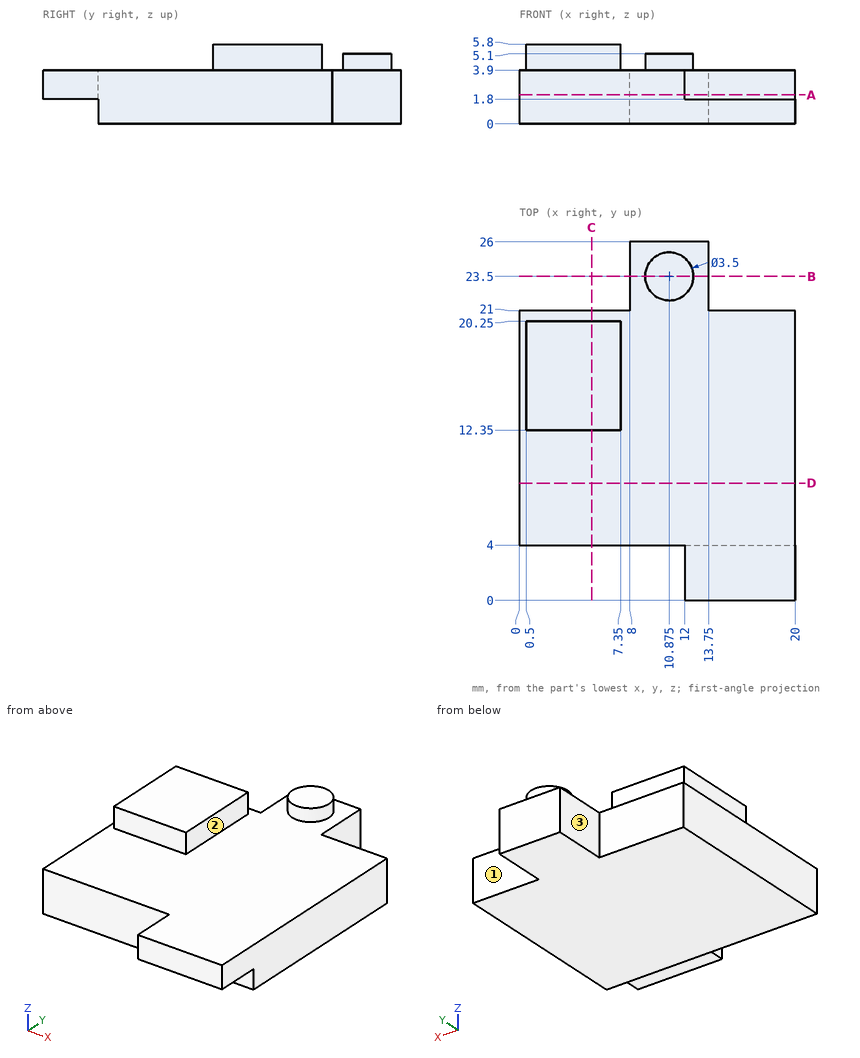
Answer from the drawing. Dimensions are ordinates in mm from the lowest x, y and z of the part. A direction names the side the tool comes from. Give positions to 0.01 mm unless a question says otherwise; leave off trailing zeros. Write each loop counter-clockwise with the first axis right and the second up, starting at its lowest first coordinate (ties: lowest second). Pieces come first, ordered by that corner, then holes. Notation, with made-up numbers: (48, 21.25) - (103, 21.25) arc R18 ccw to (103, 28.25) - close; hole circle Ø10 at (8, 80). An arc over 180 degrees is marked (long way). One line per item, written item: value. Start each with the question number.
1. For the marked faces 1, 2 and 3, determine the directions among +Z, -Z, +X, -X, +Y, -Y from which every point of the face is accessible in a straight line to the end or side of a thin tool.
2. Find section A-A (z = 2.1). Write down the section's boundary in (x, y), then the cut area to 3 significant figures.
3. Find section C-C (x = 5.25). Write down the section's boundary in (y, z), then the cut area to 3 significant figures.
4. Given pin 1 (1.2 mm diameter, centred on x = 3, z = 1.5, fed in from +Y); pin 2 (0.6 mm diameter, centred on y = 1.5, z = 2.5, fed in from -X); pin 3 (3 mm diameter, centred on x = 11.5, y = 23.5, fed in from +Z), each flat-ended and moving along its own axis, determine where each tip first touches the part or whether it passes through.
5. Consider probe 1 along Y at (x, z) = (2.75, 2.45); probe 2 along X at (y, z) = (22.25, 3.7); probe 3 along Z at (x, y) = (18, 12.5). Determine where each line is inside the solid, lowest interval first.
6. Find section D-D (y = 8.5). Write down the section's boundary in (x, z).
7. Find section B-B (y = 23.5). Write down the section's boundary in (x, z) (3 decimals), then the cut area to 3 significant figures.
Geometry results:
1. face 1: +Z, -Z, +X, +Y
1. face 2: +Z, +X, +Y, -Y
1. face 3: +Z, -Z, -X, +Y
2. outline: (0, 4) - (12, 4) - (12, 0) - (20, 0) - (20, 21) - (13.75, 21) - (13.75, 26) - (8, 26) - (8, 21) - (0, 21) - close
2. area: 401 mm2
3. outline: (4, 0) - (21, 0) - (21, 3.9) - (20.25, 3.9) - (20.25, 5.8) - (12.35, 5.8) - (12.35, 3.9) - (4, 3.9) - close
3. area: 81.3 mm2
4. pin 1: y = 21
4. pin 2: x = 12
4. pin 3: z = 5.1
5. probe 1: 4 to 21
5. probe 2: 8 to 13.75
5. probe 3: 0 to 3.9
6. outline: (0, 0) - (20, 0) - (20, 3.9) - (0, 3.9) - close
7. outline: (8, 0) - (13.75, 0) - (13.75, 3.9) - (12.625, 3.9) - (12.625, 5.1) - (9.125, 5.1) - (9.125, 3.9) - (8, 3.9) - close
7. area: 26.6 mm2
